Autodesk Fusion 360 part; units mm, degrees
sketch "Sketch1" plane through (231.1286, 0, 0) normal (-1, 0, 0) x (0, 0, 1)
  circle A0 centre (423.85, -235.9668) radius 1.5
  circle A1 centre (423.85, -270.828) radius 1.5
  line L0 (421.35, -229.9414) -> (421.35, -275.9414)
  line L1 (421.35, -275.9414) -> (426.85, -275.9414)
  line L2 (426.85, -275.9414) -> (426.85, -229.9414)
  line L3 (426.85, -229.9414) -> (421.35, -229.9414)
  circle A2 centre (423.85, -235.9668) radius 4
  dimension "d22" = 8
extrude "Extrude1" add sketch "Sketch1" along normal blind 4 contours L0 L2 L3 A2 | L0 L2 A2 | L0 L1 L2 A2
sketch "Sketch2" plane through (0, 0, 421.35) normal (0, 0, -1) x (-1, 0, 0)
  line L0 (-231.1286, -229.9414) -> (-231.1286, -275.9414)
  line L1 (-231.1286, -275.9414) -> (-227.1286, -275.9414)
  line L2 (-227.1286, -275.9414) -> (-227.1286, -229.9414)
  line L3 (-227.1286, -229.9414) -> (-231.1286, -229.9414)
  line L4 (-233.6257, -250.5312) -> (-240.5303, -250.5312)
  line L5 (-233.6257, -275.9414) -> (-240.6765, -275.9414)
  line L6 (-231.1286, -275.9414) -> (-227.1286, -275.9414)
  line L7 (-227.1286, -275.9414) -> (-227.1286, -250.5312)
  line L8 (-227.1286, -250.5312) -> (-231.1286, -250.5312)
  line L9 (-231.1286, -250.5312) -> (-231.1286, -275.9414)
extrude "Extrude2" add sketch "Sketch2" along normal blind 5 contours L0 L1 L2 L6 L7 L8 L9
sketch "Sketch3" plane through (231.1286, 0, 0) normal (1, 0, 0) x (0, 0, -1)
  circle A0 centre (-423.85, -235.9668) radius 1.5
  circle A1 centre (-423.85, -270.828) radius 1.5
  line L0 (-421.35, -229.9414) -> (-426.85, -229.9414)
  line L1 (-426.85, -229.9414) -> (-426.85, -275.9414)
  line L2 (-426.85, -275.9414) -> (-416.35, -275.9414)
  line L3 (-416.35, -275.9414) -> (-416.35, -250.5312)
  line L4 (-416.35, -250.5312) -> (-421.35, -250.5312)
  line L5 (-421.35, -250.5312) -> (-421.35, -229.9414)
  line L6 (-421.35, -275.9414) -> (-421.35, -229.9414)
extrude "Extrude3" add sketch "Sketch3" along normal blind 10 contours L2 L3 L4 L6
fillet "Fillet1" radius 3 1 edges at (229.1286, -250.5312, 421.35)
sketch "Sketch4" plane through (0, 0, 421.35) normal (0, 0, 1) x (1, 0, 0)
  line L0 (231.1286, -250.5312) -> (231.1286, -275.9414)
  line L1 (231.1286, -275.9414) -> (241.1286, -275.9414)
  line L2 (241.1286, -275.9414) -> (241.1286, -250.5312)
  line L3 (241.1286, -250.5312) -> (231.1286, -250.5312)
  circle A0 centre (237.4786, -256.5312) radius 1.6
  circle A1 centre (237.4786, -269.9414) radius 1.6
hole "Hole1" at (237.4786, -269.9414, 421.35) at (237.4786, -256.5312, 421.35) direction (0, 0, -1) diameter 3.2 depth 5 tip angle 180
move_face "OffsetFaces1" offset -0.1 1 faces at (228.462, -271.3411, 425.2595)
move_face "OffsetFaces2" offset -0.1 1 faces at (228.462, -237.0915, 422.8575)
move_face "OffsetFaces3" offset -0.05 1 faces at (232.7488, -265.2765, 421.35)
move_face "OffsetFaces4" offset -1 1 faces at (227.1286, -265.5355, 418.3695)
sketch "Sketch5" plane through (0, 0, 421.3) normal (0, 0, 1) x (1, 0, 0)
  circle A0 centre (237.4786, -269.9414) radius 1.6
  circle A1 centre (237.4786, -256.5312) radius 1.6
  line L0 (231.1286, -250.5312) -> (231.1286, -275.9414)
  line L1 (231.1286, -275.9414) -> (241.1286, -275.9414)
  line L2 (241.1286, -275.9414) -> (241.1286, -250.5312)
  line L3 (241.1286, -250.5312) -> (231.1286, -250.5312)
  circle A2 centre (237.4786, -256.5312) radius 1.6
  circle A3 centre (237.4786, -269.9414) radius 1.6
  line L4 (237.4786, -256.5312) -> (237.4786, -269.9414) construction
  line L5 (237.4786, -259.5912) -> (240.1287, -258.0612)
  line L6 (240.1287, -258.0612) -> (240.1287, -255.0012)
  line L7 (240.1287, -255.0012) -> (237.4786, -253.4712)
  line L8 (237.4786, -253.4712) -> (234.8286, -255.0012)
  line L9 (234.8286, -255.0012) -> (234.8286, -258.0612)
  line L10 (234.8286, -258.0612) -> (237.4786, -259.5912)
  line L11 (237.4786, -266.8814) -> (234.8286, -268.4114)
  line L12 (234.8286, -268.4114) -> (234.8286, -271.4714)
  line L13 (234.8286, -271.4714) -> (237.4786, -273.0014)
  line L14 (237.4786, -273.0014) -> (240.1287, -271.4714)
  line L15 (240.1287, -271.4714) -> (240.1287, -268.4114)
  line L16 (240.1287, -268.4114) -> (237.4786, -266.8814)
  dimension "d37" = 3.06
  dimension "d38" = 3.06
extrude "Extrude4" cut sketch "Sketch5" against normal blind 2.7 contours L5 L6 L7 L8 L9 L10 | L11 L12 L13 L14 L15 L16
chamfer "Chamfer1" distance 0.4 angle 45 12 edges at (234.8286, -256.5312, 421.3) (236.1536, -254.2362, 421.3) (238.8037, -254.2362, 421.3) (240.1287, -256.5312, 421.3) (238.8037, -258.8262, 421.3) (236.1536, -258.8262, 421.3) (236.1536, -267.6464, 421.3) (234.8286, -269.9414, 421.3) (236.1536, -272.2364, 421.3) (238.8037, -272.2364, 421.3) (240.1287, -269.9414, 421.3) (238.8037, -267.6464, 421.3)
Input: part model. Units: mm. Frame: model coordinates. A direction names the side the tool comes from. Round coordinates to 2 decimals unless told otherwise and drop trailing zeros. Write each loop counter-clockwise with the first axis right and the second up, starting at its lowest first coordinate (ties: lowest second). Pieces come first, ordered by that corner, then holes. Notation, with made-up numbers: M 34.25,15 L 85.25,15 A36 cw 85.25,54 Z; hole C 66,85.5 d11. An arc over 180 degrees is marked long. Write each question's results on one line, items separated by ' | '.
Q1. Section query C-C (x = 239.5). Return loops of the section in (y, z), and give its area (3 significant figures).
Results:
outline: M -275.94,416.35 L -250.53,416.35 L -250.53,421.3 L -254.18,421.3 L -254.64,420.9 L -254.64,418.6 L -258.42,418.6 L -258.42,420.9 L -258.89,421.3 L -267.59,421.3 L -268.05,420.9 L -268.05,418.6 L -271.83,418.6 L -271.83,420.9 L -272.3,421.3 L -275.94,421.3 Z | area: 105 mm^2
Q2. Section query B-B (y = -261.5). Return loops of the section in (x, z), and give its area (3 significant figures).
Results:
outline: M 228.13,416.35 L 241.13,416.35 L 241.13,421.3 L 231.13,421.3 L 231.13,426.85 L 228.13,426.85 Z | area: 81.0 mm^2
Q3. Pin query (flat end, axial travel): P1, Ø4, axis at x = 230.5, y = -246.5, coming from the -Z side; P2, Ø4, axis at x = 238, y = -271, coming from the +Z side; P3, Ø3.5, axis at y = -235.97, z = 423.85, coming from the +X side. Return the tip coordinate at first contact, or that it passes through.
Results:
P1: stops at z = 421.19 | P2: stops at z = 421.3 | P3: stops at x = 231.13
Q4. Section query D-D (z = 420). Return loops of the section in (x, y), and give its area (3 significant figures).
Results:
outline: M 228.13,-275.94 L 241.13,-275.94 L 241.13,-250.53 L 231.13,-250.53 L 231.13,-250.04 L 228.13,-250.04 Z; hole M 234.83,-271.47 L 237.48,-273 L 240.13,-271.47 L 240.13,-268.41 L 237.48,-266.88 L 234.83,-268.41 Z; hole M 234.83,-258.06 L 237.48,-259.59 L 240.13,-258.06 L 240.13,-255 L 237.48,-253.47 L 234.83,-255 Z | area: 283 mm^2
Q5. Line query: line 1 along Y through (x, z) = (229.85, 423.85); line 2 along Y through (x, z) = (235, 419.75); line 3 along X through (y, z) = (-235, 421.5). Output: solid intervals per line, ascending.
Results:
line 1: y = -275.94 to -272.43, -269.23 to -237.57, -234.37 to -229.94 | line 2: y = -275.94 to -271.57, -268.31 to -258.16, -254.9 to -250.53 | line 3: x = 228.13 to 231.13
Q6. Section query A-A (z = 423.85). Return loops of the section in (x, y), and give its area (3 significant figures).
Results:
outline: M 228.13,-275.94 L 231.13,-275.94 L 231.13,-272.43 L 228.13,-272.43 Z; M 228.13,-269.23 L 231.13,-269.23 L 231.13,-237.57 L 228.13,-237.57 Z; M 228.13,-234.37 L 231.13,-234.37 L 231.13,-229.94 L 228.13,-229.94 Z | area: 119 mm^2
Q7. Draft query along Z for faces 3 (the face through (229.65, -271.91, 422.67)), 4 (the face through (235, -263, 416.35)), 5 (the face through (236.14, -272.23, 419.77)). Return one class per face: released by +Z, released by -Z, zero draft, split by the parting line, or undercut.
Results:
face 3: undercut | face 4: released by -Z | face 5: zero draft
Q8. Access query for faces 1 (the face through (236.14, -258.82, 419.77)), 2 (the face through (230, -253, 426.85)). Directions: +Z, -Z, +X, -X, +Y, -Y. A direction counts if a zero-diameter tool reaches every point of the face in a straight line with its end or side. Return the directions, or none.
Results:
face 1: +Z | face 2: +Z, +X, -X, +Y, -Y
